The figure shows three views and two pictorial views of one solid part (mm, origin at its lowest corner). Answer the questions. A direction names the side the tool comes from. Round coordinates to 2 decimals unless told otherwise and drop trailing zeros. Order: outer loops, then holes, each group sorted by start corner. A loop starts at its lowest first (then second) coordinate and runs counter-clockwise, first axis right, second up. Notation, with made-up numbers: (36.5, 57.5) - (40.5, 57.5) arc R14 ccw to (40.5, 82.5) - close; hole circle Ø9 at (32, -2). An arc over 180 degrees is marked (long way). One line per item, written item: value. Start each with the question number.
1. Straight lines are drawn through the part: line 1 (Y direction, x = 5, z = 17); line 2 (X direction, y = 3.5, z = 11); line 3 (X direction, y = 11, z = 18). For each, find the intervals that lie inside material, in ascending order.
2. Section A-A, the plane x = 15 is taken. Give the vertices of the cut face in (y, z).
3. A flat-ended cylindrical pin translates along its axis: P1, Ø6, axis at y = 23, z = 19, coming from the +X side. Find the tip coordinate at first contact, or state that the pin passes through.
4. Section C-C, the plane y = 13 is taken. Give the vertices of the cut face in (x, z), then the cut area to 3 significant figures.
5. Section B-B, the plane z = 24.5 is taken. Give the vertices of the cut face in (x, y), then the cut area to 3 significant figures.
6. For a pull along Y with two mould halves and no side action, classify the marked faces 3, 4, 5 and 6 as released by +Y, released by -Y, zero draft, split by the parting line, or undercut.
7. A tool of negligible diameter and unlimited length cuts with its end or side. For the marked faces 1 and 2, from which of +Z, -Z, +X, -X, +Y, -Y can it reach the whole face along a straight path? Write none if from no direction.
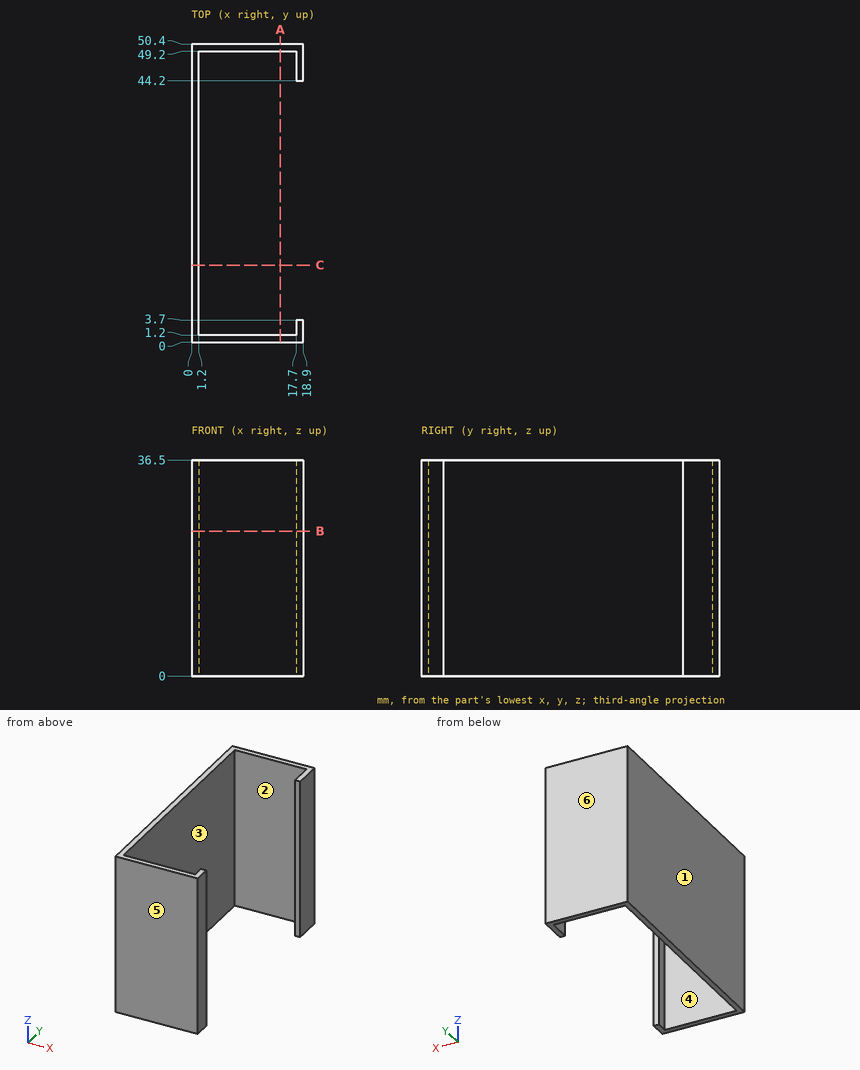
Answer list:
1. line 1: y = 0 to 1.2, 49.2 to 50.4
1. line 2: x = 0 to 1.2, 17.7 to 18.9
1. line 3: x = 0 to 1.2
2. outline: (0, 0) - (1.2, 0) - (1.2, 36.5) - (0, 36.5) - close; (49.2, 0) - (50.4, 0) - (50.4, 36.5) - (49.2, 36.5) - close
3. P1: stops at x = 1.2
4. outline: (0, 0) - (1.2, 0) - (1.2, 36.5) - (0, 36.5) - close
4. area: 43.8 mm²
5. outline: (0, 0) - (18.9, 0) - (18.9, 3.7) - (17.7, 3.7) - (17.7, 1.2) - (1.2, 1.2) - (1.2, 49.2) - (17.7, 49.2) - (17.7, 44.2) - (18.9, 44.2) - (18.9, 50.4) - (0, 50.4) - close
5. area: 112 mm²
6. face 3: undercut
6. face 4: undercut
6. face 5: released by -Y
6. face 6: released by +Y
7. face 1: +Z, -Z, -X, +Y, -Y
7. face 2: +Z, -Z
